Autodesk Inventor part; units mm, degrees
ref_plane "Work Plane1" through (-32.1046, 3.3811, 3.05) normal (0, 0, 1) x (1, 0, 0)
ref_plane "YZ Plane" through (0, 0, 0) normal (1, 0, 0) x (0, 1, 0)
ref_plane "XZ Plane" through (0, 0, 0) normal (0, 1, 0) x (-1, 0, 0)
sketch "Sketch1" plane through (0, 0, 0) normal (0, 0, 1) x (1, 0, 0)
  line L0 (-32.1046, 28.3811) -> (-17.6046, 28.3811)
  line L1 (-32.1046, 3.3811) -> (-32.1046, 28.3811)
  line L2 (-17.6046, 3.3811) -> (-32.1046, 3.3811)
  line L3 (-17.6046, 28.3811) -> (-17.6046, 3.3811)
  circle A0 centre (-21.0446, 24.002) radius 0.51
  circle A1 centre (-21.0446, 26.542) radius 0.51
  circle A2 centre (-23.5846, 26.542) radius 0.51
  circle A3 centre (-23.5846, 24.002) radius 0.51
  circle A4 centre (-26.1246, 26.542) radius 0.51
  circle A5 centre (-26.1246, 24.002) radius 0.51
  circle A6 centre (-28.6646, 26.542) radius 0.51
  circle A7 centre (-28.6646, 24.002) radius 0.51
  line L4 (-17.6046, 3.3811) -> (-17.6046, 13.3811)
  line L5 (-17.6046, 13.3811) -> (-15.6046, 13.3811)
  line L6 (-15.6046, 13.3811) -> (-15.6046, 1.3811)
  line L7 (-15.6046, 1.3811) -> (-32.1046, 1.3811)
  line L8 (-32.1046, 1.3811) -> (-34.1046, 1.3811)
  line L9 (-34.1046, 1.3811) -> (-34.1046, 13.3811)
  line L10 (-34.1046, 13.3811) -> (-32.1046, 13.3811)
  point P0 (0, 0)
  dimension "d0" = 10
  dimension "d1" = 2
  dimension "d2" = 90
  dimension "d3" = 12
  dimension "d4" = 90
  dimension "d5" = 2
  dimension "d6" = 12
ref_plane "Work Plane1" through (-32.1046, 3.3811, 3.05) normal (0, 0, 1) x (1, 0, 0)
extrude "Extrusion1" add sketch "Sketch1" along normal up to surface (3.05 mm away) contours L1 L2 L3 L5 L6 L7 L8 L9 L10
sketch "Sketch2" plane through (-34.1046, 1.3811, 3.05) normal (0, 0, 1) x (1, 0, 0)
  line L0 (16.5, 12) -> (18.5, 12)
  line L1 (18.5, 12) -> (0, 12)
  line L2 (0, 12) -> (0, 0)
  line L3 (0, 0) -> (18.5, 0)
  line L4 (18.5, 0) -> (18.5, 12)
  point P0 (34.1046, -1.3811)
extrude "Extrusion2" add sketch "Sketch2" along normal blind 2
sketch "Sketch3" plane through (-34.1046, 1.3811, 0) normal (0, -1, 0) x (1, 0, 0)
  line L0 (16.5, 0) -> (2, 0)
  line L1 (9.25, 0) -> (6.25, 0)
  line L2 (6.25, 0) -> (6.25, 3)
  line L3 (6.25, 3) -> (9.25, 3)
  line L4 (9.25, 3) -> (9.25, 0)
  line L5 (9.25, 3) -> (12.25, 3)
  line L6 (12.25, 3) -> (12.25, 0)
  line L7 (12.25, 0) -> (9.25, 0)
  line L8 (9.25, 0) -> (9.25, 3)
  point P0 (34.1046, 0)
  dimension "d11" = 3
  dimension "d12" = 3
  dimension "d13" = 3
extrude "Extrusion3" add sketch "Sketch3" along normal blind 6
fillet "Fillet1" radius 1.5 8 edges at (-27.8546, -4.6189, 1.5) (-21.8546, -4.6189, 1.5) (-24.8546, 1.3811, 3) (-27.8546, 1.3811, 1.5) (-21.8546, 1.3811, 1.5) (-27.8546, -1.6189, 3) (-21.8546, -1.6189, 3) (-24.8546, -4.6189, 3)
sketch "Sketch4" plane through (-26.3546, -3.1189, 3) normal (0, 0, 1) x (1, 0, 0)
  line L0 (0, 3) -> (3, 3)
  line L1 (3, 3) -> (3, 0)
  circle A0 centre (1.5, 1.5) radius 1.5
  point P0 (26.3546, 3.1189)
  dimension "d17" = 3
extrude "Extrusion4" cut sketch "Sketch4" against normal blind 6 contours A0
fillet "Fillet2" radius 0.5 11 edges at (-15.6046, 1.3811, 2.525) (-34.1046, 1.3811, 2.525) (-24.8546, 1.3811, 5.05) (-34.1046, 13.3811, 2.525) (-24.8546, 13.3811, 5.05) (-15.6046, 13.3811, 2.525) (-24.8546, 13.3811, 3.05) (-17.6046, 13.3811, 1.525) (-32.1046, 13.3811, 1.525) (-34.1046, 7.3811, 5.05) (-15.6046, 7.3811, 5.05)
properties part number "soporte esp1"
Part model, mm, in its own coordinate system. A direction names the side the tool comes from. Round coordinates to 2 decimals unless told otherwise and drop trailing zeros. Order: outer loops, then holes, each group sorted by start corner. A loop starts at its lowest first (then second) coordinate and runs counter-clockwise, first axis right, second up. Notation, with made-up numbers: M 47.25,88.25 L 62.25,88.25 A23 cw 62.25,101.25 Z; hole C -22,56.25 d9. An arc over 180 degrees is marked long. Answer in a Markdown table with one row per item. Add a question column.
Q1. Cut at B-B on y = 11. Give the cut face in (x, z), and give its area (3 significant figures).
Q2. Cut at C-C on x = -19.75. Give the cut face in (y, z), and give its area (3 significant figures).
Q3. Wall check: L1, parallel to X at y = -1.5, z = 0.7; L2, parallel to X at y = 11, z = 1.2; L3, parallel to Z at x = -28.25, y = 9.75. Give the ranges that are in metal, low to high. Write a range as from..to.
Q4. Mould opens along X. For faces 1 (the face through (-23.7, -2.8, 3)), 2 (the face through (-21.855, -2, 1)), 3 (the face through (-32.105, 8, 2)) say: +X half, -X half, draft (parallel to the pull), parting line (faces both ways), or undercut.
Q5. Cut at A-A on y = -0.5. Give the cut face in (x, z), and give its area (3 significant figures).
Q6. Pin check, flat tips, straight feed: pin 1 (1.2 mm diameter, centred on x = -25.5, y = -2, fed in from +Z); pin 2 (1.2 mm diameter, centred on y = -2.5, z = 1, fed in from +X); pin 3 (1.4 mm diameter, centred on x = -28, z = 3.5, fed in from -Y); pin 4 (1.5 mm diameter, centred on x = -29.5, z = 1.5, fed in from +Y). Stop position of each tip, or through.
Q7. 3-axis set-ups, long thin cutter, end or side, ignore diameter. For faces 4 (the face through (-27.404, -1.64, 2.572)), 5 (the face through (-22.282, -1.64, 2.549)), 6 (the face through (-26.1, -2.8, 3)), 7 (the face through (-21, 1.381, 4)): which of +Z, -Z, +X, -X, +Y, -Y reach the whole face in a straight line?
Q8. Cut at D-D on y = -2.5. Give the cut face in (x, z).
Established:
| question | item | result |
|---|---|---|
| 1 | outline | M -34.1,0 L -32.1,0 L -32.1,3.05 L -17.6,3.05 L -17.6,0 L -15.6,0 L -15.6,4.55 A0.5 ccw -16.1,5.05 L -33.6,5.05 A0.5 ccw -34.1,4.55 Z |
| 1 | area | 49.1 mm2 |
| 2 | outline | M 1.38,0 L 3.38,0 L 3.38,3.05 L 12.88,3.05 A0.5 ccw 13.38,3.55 L 13.38,4.55 A0.5 ccw 12.88,5.05 L 1.88,5.05 A0.5 ccw 1.38,4.55 Z |
| 2 | area | 29.9 mm2 |
| 3 | L1 | x = -27.85..-26.35, -23.36..-21.85 |
| 3 | L2 | x = -34.1..-32.1, -17.6..-15.6 |
| 3 | L3 | z = 3.05..5.05 |
| 4 | face 1 | draft |
| 4 | face 2 | +X half |
| 4 | face 3 | undercut |
| 5 | outline | M -27.85,0 L -25.85,0 L -25.85,3 L -26.35,3 A1.5 ccw -27.85,1.5 Z; M -23.86,0 L -21.85,0 L -21.85,1.5 A1.5 ccw -23.35,3 L -23.86,3 Z |
| 5 | area | 11.0 mm2 |
| 6 | pin 1 | passes through |
| 6 | pin 2 | stops at x = -21.85 |
| 6 | pin 3 | stops at y = 0.89 |
| 6 | pin 4 | stops at y = 3.38 |
| 7 | face 4 | +Z, -X, -Y |
| 7 | face 5 | +Z, +X, -Y |
| 7 | face 6 | +Z, +X, -X, -Y |
| 7 | face 7 | +Z, -Y |
| 8 | outline | M -27.85,0 L -26.07,0 L -26.07,3 L -26.35,3 A1.5 ccw -27.85,1.5 Z; M -23.64,0 L -21.85,0 L -21.85,1.5 A1.5 ccw -23.35,3 L -23.64,3 Z |
